Could you check a few things on this model? Use its own coordinates, in mm. Give positions to 0.01 mm unless a question says otherwise; leave off trailing zeros. Loops run counter-clockwise (first coordinate to the right, second up) from the corner with the lowest first, then second, coordinate; pieces in that order, holes last. Notation, with made-up numbers: M 79.5,-20.75 L 91.5,-20.75 A16 ccw 91.5,-16.75 Z; hole C 19.25,57.5 d6. An arc over 180 degrees is marked long. Answer in a Markdown table with one row per item. Add a question column.
```python
from build123d import *

# Parameters (mm, degrees)
ESQUISSE1_W             = 41.2
ESQUISSE1_H             = 25.2
BOSS_EXTRU_1_DEPTH      = 12
ESQUISSE2_R             = 2.2
ENL_V_MAT_EXTRU_1_DEPTH = 12


with BuildPart() as part:
    # Esquisse1 → Boss.-Extru.1 (new body)
    with BuildSketch(Plane.XY):
        Rectangle(ESQUISSE1_W, ESQUISSE1_H)
    extrude(amount=BOSS_EXTRU_1_DEPTH)

    # Esquisse2 → Enlèv. mat.-Extru.1 (cut)
    with BuildSketch(Plane.XY):
        with Locations((8, 0)):
            Circle(ESQUISSE2_R)
        with Locations((-8, 0)):
            Circle(ESQUISSE2_R)
    extrude(amount=ENL_V_MAT_EXTRU_1_DEPTH, mode=Mode.SUBTRACT)


solid = part.part
```
Item 1: Suppose I cut it at A-A (x = -8). List the corners of the cut face in (y, z) for me, then the cut area to 3 significant figures.
Item 2: Suppose I cut it at C-C (z = 7.75). List the corners of the cut face in (x, y) for me.
Item 3: Suppose I cut it at B-B (y = 0). List the corners of the cut face in (x, z) for me.
Item 4: If we mould it in two halves opening along Y, with no side actions, what happens to faces 1 (the face through (0, 12.6, 6)), 2 (the face through (20.6, 0, 6)), 3 (the face through (-5.9, 0.66, 5.92))? For each: +Y half, -Y half, draft (parallel to the pull), parting line (faces both ways), or undercut.
Item 5: I need wall thicknesses on L1, parallel to X at y = -1, z = 1.5; L2, parallel to Y at x = -8, z = 8.75; L3, parallel to X at y = 1.5, z = 1.75. Which ranges of each line are inside material? Lowest first, please.
Values found:
| question | item | result |
|---|---|---|
| 1 | outline | M -12.6,0 L -2.2,0 L -2.2,12 L -12.6,12 Z; M 2.2,0 L 12.6,0 L 12.6,12 L 2.2,12 Z |
| 1 | area | 250 mm² |
| 2 | outline | M -20.6,-12.6 L 20.6,-12.6 L 20.6,12.6 L -20.6,12.6 Z; hole C -8,0 d4.4; hole C 8,0 d4.4 |
| 3 | outline | M -20.6,0 L -10.2,0 L -10.2,12 L -20.6,12 Z; M -5.8,0 L 5.8,0 L 5.8,12 L -5.8,12 Z; M 10.2,0 L 20.6,0 L 20.6,12 L 10.2,12 Z |
| 4 | face 1 | +Y half |
| 4 | face 2 | draft |
| 4 | face 3 | undercut |
| 5 | L1 | -20.6 to -9.96, -6.04 to 6.04, 9.96 to 20.6 |
| 5 | L2 | -12.6 to -2.2, 2.2 to 12.6 |
| 5 | L3 | -20.6 to -9.61, -6.39 to 6.39, 9.61 to 20.6 |
